Autodesk Inventor part; units mm, degrees
ref_plane "Arbeitsebene1" through (0, 0, 0) normal (-0.7071, 0.7071, 0) x (0, 0, 1)
ref_plane "YZ Plane" through (0, 0, 0) normal (1, 0, 0) x (0, 1, 0)
ref_plane "XY Plane" through (0, 0, 0) normal (0, 0, 1) x (1, 0, 0)
sketch "Skizze1" plane through (0, 0, 0) normal (0, 0, 1) x (1, 0, 0)
  circle A0 centre (0, 0) radius 25.1
  circle A1 centre (0, 0) radius 30
  line L0 (-42.5, -42.5) -> (42.5, -42.5)
  line L1 (42.5, -42.5) -> (42.5, 42.5)
  line L2 (42.5, 42.5) -> (-42.5, 42.5)
  line L3 (-42.5, 42.5) -> (-42.5, -42.5)
  line L4 (-42.5, -42.5) -> (42.5, 42.5) construction
  line L5 (42.5, -42.5) -> (-42.5, 42.5) construction
  dimension "d0" = 50.2
  dimension "d2" = 60
  dimension "d25" = 85
  dimension "d26" = 85
extrude "Extrusion1" add sketch "Skizze1" against normal blind 7 contours A1 | L3 L2 L1 L0
extrude "Extrusion2" add sketch "Skizze1" along normal blind 35 contours A1
ref_plane "Arbeitsebene1" through (0, 0, 0) normal (-0.7071, 0.7071, 0) x (0, 0, 1)
sketch "Skizze2" plane through (0, 0, 0) normal (-0.7071, 0.7071, 0) x (-0.7071, -0.7071, 0)
  line L0 (25.1, 35) -> (30, 35)
  line L1 (30, 35) -> (30, 0)
  line L2 (-30, 0) -> (-30, 35)
  line L3 (-30, 35) -> (-25.1, 35)
  line L4 (-30, 35) -> (-30, 0)
  line L5 (-30, 5) -> (-30, 35)
  line L6 (0, -15.4) -> (0, 43.4)
  line L7 (25.1, -7) -> (25.1, 35)
  line L8 (-25.1, 35) -> (-25.1, -7)
  line L9 (-60.1041, 0) -> (-30, 0)
  line L10 (30, 0) -> (60.1041, 0)
  line L11 (-60.1041, -7) -> (-60.1041, 0)
  line L12 (-25.1, -7) -> (-60.1041, -7)
  line L13 (60.1041, 0) -> (60.1041, -7)
  line L14 (60.1041, -7) -> (25.1, -7)
  line L15 (-30, 35) -> (-55, 0)
  line L16 (-30, 0) -> (-55, 0)
  line L17 (-30, 0) -> (-25.1, 0)
  line L18 (-25.1, 0) -> (-25.1, 35)
  line L19 (-25.1, 35) -> (-30, 35)
  line L20 (-30, 35) -> (-30, 0)
  point P0 (0, 0)
  point P1 (-42.5, -7)
  point P2 (0, 0)
  dimension "d28" = 25
extrude "Extrusion3" add sketch "Skizze2" along normal mid plane 5 contours L9 L15 L2 | L2 L3 L8 L17
pattern_circular "Runde Anordnung1" count 4 over 360 about axis through (0, 0, -10) along (0, 0, 1) of "Extrusion3"
sketch "Skizze3" plane through (0, 0, 0) normal (0, 0, 1) x (1, 0, 0)
  arc A0 (-19.3717, -22.9072) -> (19.3717, -22.9072) centre (0, 0) ccw
  arc A1 (-22.9072, 19.3717) -> (-22.9072, -19.3717) centre (0, 0) ccw
  arc A2 (22.9072, -19.3717) -> (22.9072, 19.3717) centre (0, 0) ccw
  line L0 (-42.5, 42.5) -> (-42.5, -42.5)
  circle A3 centre (0, 0) radius 42.5 construction
  circle A4 centre (0, 0) radius 30 construction
  circle A5 centre (0, 0) radius 36.25
  point P0 (-36.25, 0)
  dimension "d31" = 72.5
  dimension "d29" = 60
  dimension "d30" = 85
hole "Bohrung2" at (-36.25, 0, 0) direction (0, 0, -1) diameter 5.5 end through all countersink diameter 10.4 countersink angle 90
pattern_circular "Runde Anordnung3" count 4 over 360 about axis through (0, 0, -10) along (0, 0, 1) of "Bohrung2"
equation "\"d0\" = ht_diameter + 2 * gap_fit"
equation "\"kg_thickness\" = 4.9"
equation "\"ht_thickness\" = 1.9"
equation "\"case_thickness\" = 18"
equation "\"gap_fit\" = 0.1"
equation "\"gap_slide\" = 0.2"
equation "\"gap_air\" = 1"
equation "\"bore_diameter\" = 73"
equation "\"mdf_thickness\" = 6"
equation "\"tape_thickness\" = 3"
equation "\"tape_width\" = 15"
equation "\"inner_thickness\" = 15"
equation "\"inner_depth\" = 255"
properties part number "Zyklon_Flansch"
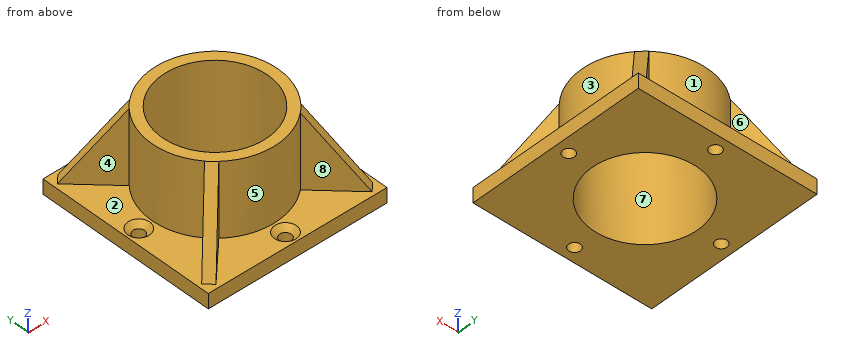
Model file for the job. Use its own axes, mm. Face numbers are marked on the shaded views. A direction names the side the tool comes from. Coordinates: 2 decimals unless noted, no trailing zeros. Loops run counter-clockwise (first coordinate to the right, second up) from the corner with the lowest first, then second, coordinate; pieces in that order, holes last. Notation, with made-up numbers: (-2, 39.5) - (30, 39.5) arc R27 ccw to (30, 68.5) - close; hole circle Ø3 at (-6.5, -5). An arc over 180 degrees is marked (long way). Write item = value, one per line. Start each with the question number.
Item 1: Saw through at A-A, the plane x = 0. List the corners of the cut face in (y, z), then the cut area to 3 significant figures.
Item 2: 3-axis set-ups, long thin cutter, end or side, ignore diameter. For the marked faces 1, 2, 3, 4 and 5: which of +Z, -Z, +X, -X, +Y, -Y reach the whole face in a straight line?
Item 3: Saw through at D-D, the plane z = 8.5. List the corners of the cut face in (x, y), then the cut area to 3 significant figures.
Item 4: Pull direction Y, two halves, no side cores. Call the marked faces 6, 7 and 8: +Y half, -Y half, draft (parallel to the pull), parting line (faces both ways), or undercut.
Item 5: Saw through at C-C, the plane x = 12. List the corners of the cut face in (y, z), then the cut area to 3 significant figures.
Item 6: Wall check: probe 1 along Y at (x, z) = (0, -6); probe 2 along Y at (x, z) = (0, 16.5). Give the ranges that are in metal, low to high. Write a range as [from, to].
Item 7: Drop flat-ended pins along their axis: pin 1 Ø7 at (x, y) = (0, 36.25) entering from +Z; pin 2 Ø6 at (x, y) = (-27.5, 30) entering from +Z; pin 3 Ø2 at (y, z) = (20, 7) entering from -X. Give the stop position or say it passes through.
Answers:
q1.outline = (-42.5, -7) - (-39, -7) - (-39, -2.45) - (-41.45, 0) - (-42.5, 0) - close; (-33.5, -7) - (-25.1, -7) - (-25.1, 35) - (-30, 35) - (-30, 0) - (-31.05, 0) - (-33.5, -2.45) - close; (25.1, -7) - (33.5, -7) - (33.5, -2.45) - (31.05, 0) - (30, 0) - (30, 35) - (25.1, 35) - close; (39, -7) - (42.5, -7) - (42.5, 0) - (41.45, 0) - (39, -2.45) - close
q1.area = 498 mm2
q2.face_1 = +Z, +Y
q2.face_2 = +Z
q2.face_3 = +Z, +X
q2.face_4 = +Z, -X
q2.face_5 = +Z, -Y
q3.outline = (-36.37, -32.83) - (-32.83, -36.37) - (-19.37, -22.91) arc R30 ccw to (19.37, -22.91) - (32.83, -36.37) - (36.37, -32.83) - (22.91, -19.37) arc R30 ccw to (22.91, 19.37) - (36.37, 32.83) - (32.83, 36.37) - (19.37, 22.91) arc R30 ccw to (-19.37, 22.91) - (-32.83, 36.37) - (-36.37, 32.83) - (-22.91, 19.37) arc R30 ccw to (-22.91, -19.37) - close; hole circle Ø50.2 at (0, 0)
q3.area = 1,230 mm2
q4.face_6 = +Y half
q4.face_7 = undercut
q4.face_8 = -Y half
q5.outline = (-42.5, -7) - (-22.05, -7) - (-22.05, 35) - (-27.5, 35) - (-27.5, 0) - (-42.5, 0) - close; (22.05, -7) - (42.5, -7) - (42.5, 0) - (27.5, 0) - (27.5, 35) - (22.05, 35) - close
q5.area = 668 mm2
q6.probe_1 = [-42.5, -39], [-33.5, -25.1], [25.1, 33.5], [39, 42.5]
q6.probe_2 = [-30, -25.1], [25.1, 30]
q7.pin_1 = -1.7
q7.pin_2 = 24.28
q7.pin_3 = -24.54
